```python
from build123d import *

# Parameters (mm, degrees)
BOSS_EXTRUDE1_DEPTH = 25.654
SKETCH2_W           = 20.6502
SKETCH2_H           = 12.3952
CUT_EXTRUDE1_DEPTH  = 63.010623853
SKETCH3_W           = 42.037
SKETCH3_H           = 20.6502
CUT_EXTRUDE2_DEPTH  = 62.078275718
CUT_EXTRUDE3_DEPTH  = 5.08
SKETCH5_R           = 1.0795
CUT_EXTRUDE4_DEPTH  = 62.078275718
SKETCH6_R           = 1.7145
CUT_EXTRUDE5_DEPTH  = 63.010623853
SKETCH7_W           = 13.199565881
SKETCH7_H           = 28.375595839
SKETCH7_W_2         = 9.485915606
CUT_EXTRUDE6_DEPTH  = 63.010623853
SKETCH8_W           = 38.481
SKETCH8_H           = 14.6304
CUT_EXTRUDE7_DEPTH  = 59.330512418
SKETCH9_W           = 1.4732
SKETCH9_H           = 5.0038
CUT_EXTRUDE8_DEPTH  = 2.54


with BuildPart() as part:
    # Sketch1 → Boss-Extrude1 (new body)
    with BuildSketch(Plane.XY):
        with BuildLine():
            Line((0, 0), (54.0258, 0))
            Line((54.0258, 0), (54.0258, 3.9878))
            Line((54.0258, 3.9878), (51.176616962, 11.038320738))
            ThreePointArc((51.176616962, 11.038320738), (51.065947457, 11.411860999), (51.0286, 11.799656349))
            Line((51.0286, 11.799656349), (51.0286, 15.113))
            Line((51.0286, 15.113), (49.7586, 16.383))
            Line((49.7586, 16.383), (11.2776, 16.383))
            Line((11.2776, 16.383), (10.0076, 15.113))
            Line((10.0076, 15.113), (10.0076, 12.427861529))
            ThreePointArc((10.0076, 12.427861529), (9.790474401, 11.513938717), (9.185498713, 10.795326965))
            Line((9.185498713, 10.795326965), (0, 3.9878))
            Line((0, 3.9878), (0, 0))
        make_face()
    extrude(amount=-BOSS_EXTRUDE1_DEPTH)

    # Sketch2 → Cut-Extrude1 (cut, through all)
    with BuildSketch(Plane(origin=(54.0258, 0, 0), x_dir=(0, 0, -1), z_dir=(1, 0, 0))):
        with Locations((15.3289, 10.1854)):
            Rectangle(SKETCH2_W, SKETCH2_H)
    extrude(amount=-CUT_EXTRUDE1_DEPTH, mode=Mode.SUBTRACT)

    # Sketch3 → Cut-Extrude2 (cut, through all)
    with BuildSketch(Plane(origin=(0, 3.9878, 0), x_dir=(1, 0, 0), z_dir=(0, 1, 0))):
        with Locations((27.0129, 15.3289)):
            Rectangle(SKETCH3_W, SKETCH3_H)
    extrude(amount=-CUT_EXTRUDE2_DEPTH, mode=Mode.SUBTRACT)

    # Sketch4 → Cut-Extrude3 (cut)
    with BuildSketch(Plane.XY):
        with BuildLine():
            Line((6.901956547, 3.937), (10.414, 3.937))
            ThreePointArc((10.414, 3.937), (11.473670222, 4.375929778), (11.9126, 5.4356))
            Line((11.9126, 5.4356), (11.9126, 8.038434234))
            ThreePointArc((11.9126, 8.038434234), (11.088018074, 9.376904105), (9.521699699, 9.242428475))
            Line((9.521699699, 9.242428475), (6.009656246, 6.639594241))
            ThreePointArc((6.009656246, 6.639594241), (5.478912674, 4.965761629), (6.901956547, 3.937))
        make_face()
        with BuildLine():
            Line((47.752, 13.9446), (42.6212, 13.9446))
            ThreePointArc((42.6212, 13.9446), (41.561529778, 13.505670222), (41.1226, 12.446))
            Line((41.1226, 12.446), (41.1226, 5.4356))
            ThreePointArc((41.1226, 5.4356), (41.561529778, 4.375929778), (42.6212, 3.937))
            Line((42.6212, 3.937), (47.752, 3.937))
            ThreePointArc((47.752, 3.937), (48.811670222, 4.375929778), (49.2506, 5.4356))
            Line((49.2506, 5.4356), (49.2506, 12.446))
            ThreePointArc((49.2506, 12.446), (48.811670222, 13.505670222), (47.752, 13.9446))
        make_face()
        with BuildLine():
            Line((13.3096, 12.446), (13.3096, 5.4356))
            ThreePointArc((13.3096, 5.4356), (13.748529778, 4.375929778), (14.8082, 3.937))
            Line((14.8082, 3.937), (19.939, 3.937))
            ThreePointArc((19.939, 3.937), (20.998670222, 4.375929778), (21.4376, 5.4356))
            Line((21.4376, 5.4356), (21.4376, 12.446))
            ThreePointArc((21.4376, 12.446), (20.998670222, 13.505670222), (19.939, 13.9446))
            Line((19.939, 13.9446), (14.8082, 13.9446))
            ThreePointArc((14.8082, 13.9446), (13.748529778, 13.505670222), (13.3096, 12.446))
        make_face()
        with BuildLine():
            Line((22.8346, 12.446), (22.8346, 5.4356))
            ThreePointArc((22.8346, 5.4356), (23.273529778, 4.375929778), (24.3332, 3.937))
            Line((24.3332, 3.937), (38.227, 3.937))
            ThreePointArc((38.227, 3.937), (39.286670222, 4.375929778), (39.7256, 5.4356))
            Line((39.7256, 5.4356), (39.7256, 12.446))
            ThreePointArc((39.7256, 12.446), (39.286670222, 13.505670222), (38.227, 13.9446))
            Line((38.227, 13.9446), (24.3332, 13.9446))
            ThreePointArc((24.3332, 13.9446), (23.273529778, 13.505670222), (22.8346, 12.446))
        make_face()
    extrude(amount=-CUT_EXTRUDE3_DEPTH, mode=Mode.SUBTRACT)

    # Sketch5 → Cut-Extrude4 (cut, through all)
    with BuildSketch(Plane(origin=(0, 3.9878, 0), x_dir=(1, 0, 0), z_dir=(0, 1, 0))):
        with Locations(Location((51.0286, 21.336, 0), (0, 0, 270))):
            Circle(SKETCH5_R)
        with Locations(Location((51.0286, 11.3538, 0), (0, 0, 270))):
            Circle(SKETCH5_R)
        with Locations(Location((2.9972, 11.3538, 0), (0, 0, 90))):
            Circle(SKETCH5_R)
        with Locations(Location((2.9972, 21.336, 0), (0, 0, 90))):
            Circle(SKETCH5_R)
    extrude(amount=-CUT_EXTRUDE4_DEPTH, mode=Mode.SUBTRACT)

    # Sketch6 → Cut-Extrude5 (cut, through all)
    with BuildSketch(Plane.XZ):
        with Locations(Location((45.2501, -2.5019, 0), (0, 0, 270))):
            Circle(SKETCH6_R)
        with Locations(Location((17.2593, -2.5019, 0), (0, 0, 270))):
            Circle(SKETCH6_R)
    extrude(amount=-CUT_EXTRUDE5_DEPTH, mode=Mode.SUBTRACT)

    # Sketch7 → Cut-Extrude6 (cut, through all)
    with BuildSketch(Plane(origin=(0, 16.383, 0), x_dir=(1, 0, 0), z_dir=(0, 1, 0))):
        with Locations((4.67781706, 13.121352654)):
            Rectangle(SKETCH7_W, SKETCH7_H)
        with Locations((54.501557803, 13.121352654)):
            Rectangle(SKETCH7_W_2, SKETCH7_H)
    extrude(amount=-CUT_EXTRUDE6_DEPTH, mode=Mode.SUBTRACT)

    # Sketch8 → Cut-Extrude7 (cut, through all)
    with BuildSketch(Plane.XY):
        with Locations((30.5181, 7.3152)):
            Rectangle(SKETCH8_W, SKETCH8_H)
    extrude(amount=-CUT_EXTRUDE7_DEPTH, mode=Mode.SUBTRACT)

    # Sketch9 → Cut-Extrude8 (cut)
    with BuildSketch(Plane(origin=(0, 16.383, 0), x_dir=(1, 0, 0), z_dir=(0, 1, 0))):
        with Locations((12.0142, 2.5019)):
            Rectangle(SKETCH9_W, SKETCH9_H)
    extrude(amount=-CUT_EXTRUDE8_DEPTH, mode=Mode.SUBTRACT)


solid = part.part
```
The listing builds one solid part. Answer for the finished solid, in the listing's coordinates (mm). Coordinates: 2 decimals unless noted, no trailing zeros. Loops run counter-clockwise (first coordinate to the right, second up) from the corner with the lowest first, then second, coordinate; pieces in that order, holes last. Notation, with made-up numbers: M -11.5,16 L 5.5,16 A26 cw 5.5,49 Z; hole C 19,-4 d9. An arc over 180 degrees is marked long. Answer as CSV lines item,"result". Start each with the question number.
(1) The mould has two halves that part along X. Classify faces 1 (the cylindrical face through (43.729, 15.494, -3.293)), 2 (the flat face through (32, 16.383, -2)), 3 (the cylindrical face through (15.738, 15.494, -3.293)), 4 (the flat face through (49.759, 16, -2)): pulls with the +X half, pulls with the -X half, needs draft (parallel to the pull), parting line crosses it, or undercut.
(2) Find the intervals of material crossed by L1, parallel to X at y = 14.8, z = -3.15; L2, parallel to X at y = 15.55, z = -3.95; L3, parallel to Z at x = 46.5, y = 16.05, in increasing order. Write a range as [from, to].
(3) The part is cut by section B-B (x = 46). Give the vertices of the cut face in (y, z).
(4) The part is cut by section A-A (z = -2.6). Give the vertices of the cut face in (x, y), and give its area (3 significant figures).
(5) The part is cut by section C-C (y = 15.95). Give the vertices of the cut face in (x, z).
Determined:
1,face 1,"undercut"
1,face 2,"needs draft"
1,face 3,"undercut"
1,face 4,"pulls with the +X half"
2,L1,"[12.75, 15.67], [18.85, 43.66], [46.84, 49.76]"
2,L2,"[12.75, 16.34], [18.18, 44.33], [46.17, 49.76]"
2,L3,"[-5, -3.68], [-1.33, 0]"
3,outline,"M 14.63,-5 L 16.38,-5 L 16.38,-4.04 L 14.63,-4.04 Z; M 14.63,-0.96 L 16.38,-0.96 L 16.38,0 L 14.63,0 Z"
4,outline,"M 12.75,14.63 L 15.55,14.63 L 15.55,16.38 L 12.75,16.38 Z; M 18.97,14.63 L 43.54,14.63 L 43.54,16.38 L 18.97,16.38 Z; M 46.96,14.63 L 49.76,14.63 L 49.76,16.38 L 46.96,16.38 Z"
4,area,"52.9 mm2"
5,outline,"M 12.75,-5 L 49.76,-5 L 49.76,0 L 12.75,0 Z; hole C 17.26,-2.5 d3.43; hole C 45.25,-2.5 d3.43"
